The listing builds one solid part. Answer for the finished solid, in the listing's coordinates (mm). Round coordinates to 2 decimals unless told otherwise and drop trailing zeros. Order: outer loops, then holes, each group sorted by start corner. A loop starts at its lowest first (then second) coordinate and runs counter-clockwise, first axis right, second up. Notation, with made-up numbers: (13, 11) -> (36, 11) arc R8 ccw to (36, 17) -> close; hole circle Ø1 at (71.5, -1.75). An arc over 180 degrees is marked (long way). Return JSON: item names as keys, results as strings. Group by question number.
(1) Consider line 1 (X direction, y = 31.5, z = -1); line 2 (Y direction, x = 0.5, z = -31); line 3 (Y direction, x = 16.5, z = -3). Determine where each line is inside the solid, lowest interval first. Write a range as [from, to].
(2) The part is cut by section A-A (x = -11). Determine the outline of the cut face in (y, z), plus the area to 3 significant figures.
(3) The part is cut by section B-B (y = 24). Determine the outline of the cut face in (x, z), plus the area to 3 significant figures.
(4) The part is cut by section C-C (z = 33.5). Determine the outline of the cut face in (x, y).
(5) The part is cut by section D-D (y = -13.5). Determine the outline of the cut face in (x, z), plus the area to 3 significant figures.
(6) Each of these flat-tipped pins is pushed along its axis until it touches: pin 1 (24 mm diameter, centred on x = 1.5, z = 1.5, fed in from +Y); pin 2 (4 mm diameter, centred on x = -15.5, y = -4, fed in from -Z); pin 3 (1.5 mm diameter, centred on y = 39.5, z = 76, fed in from +X). Where does it stop, or does it pass through?
Autodesk Inventor part; units mm, degrees
ref_plane "Plano de trabalho1" through (0, 31, -25) normal (0, 0, 1) x (1, 0, 0)
ref_plane "YZ Plane" through (0, 0, 0) normal (1, 0, 0) x (0, 1, 0)
ref_plane "XZ Plane" through (0, 0, 0) normal (0, 1, 0) x (-1, 0, 0)
sketch "Esboço1" plane through (0, 0, 0) normal (0, 1, 0) x (-1, 0, 0)
  circle A0 centre (0, 0) radius 15
  dimension "d0" = 30
extrude "Extrusão1" add sketch "Esboço1" along normal blind 30
sketch "Esboço2" plane through (0, 30, 0) normal (0, 1, 0) x (1, 0, 0)
  circle A0 centre (0, 0) radius 2
  dimension "d3" = 4
extrude "Extrusão2" add sketch "Esboço2" along normal blind 1
sketch "Esboço3" plane through (0, 31, 0) normal (0, 1, 0) x (1, 0, 0)
  circle A0 centre (0, 0) radius 25
  dimension "d6" = 50
extrude "Extrusão3" add sketch "Esboço3" along normal blind 10
ref_plane "Plano de trabalho1" through (0, 31, -25) normal (0, 0, 1) x (1, 0, 0)
sketch "Esboço4" plane through (0, 31, -25) normal (0, 0, 1) x (1, 0, 0)
  line L0 (2, 0) -> (-2, 0)
  line L1 (0, 0) -> (0, 10)
  line L2 (25, 10) -> (-25, 10)
  circle A0 centre (0, 5) radius 2.5
  point P0 (0, -31)
  dimension "d9" = 5
extrude "Extrusão4" add sketch "Esboço4" along normal blind 80 and the other way blind 70
sketch "Esboço5" plane through (0, 0, 0) normal (1, 0, 0) x (0, 1, 0)
  line L0 (33.5, -95) -> (38.5, -95)
  line L1 (36, -95) -> (36, -105)
  line L2 (36, -95) -> (46, -95) construction
  line L3 (36, -105) -> (33.5, -95)
  line L4 (36, -95) -> (33.5, -95)
  point P0 (0, 0)
  dimension "d14" = 10
  dimension "d15" = 90
revolve "Revolução1" add sketch "Esboço5" angle 360 about axis through (0, 36, -95) along (0, 0, -1)
sketch "Esboço6" plane through (0, 0, 0) normal (1, 0, 0) x (0, 1, 0)
  line L0 (38.5, 55) -> (33.5, 55)
  line L1 (33.5, 25) -> (33.5, 55)
  line L2 (38.5, 25) -> (38.5, 55)
  line L3 (33.5, 55) -> (38.5, 55)
  line L4 (6, 113) -> (6, 101.4068)
  line L5 (6.7336, 98.7996) -> (33.5, 55)
  line L6 (8, 115) -> (84, 115)
  line L7 (86, 113) -> (86, 99.2532)
  line L8 (84.312, 95.5075) -> (38.5, 55)
  arc A0 (84.312, 95.5075) -> (86, 99.2532) centre (81, 99.2532) ccw
  arc A1 (6, 101.4068) -> (6.7336, 98.7996) centre (11, 101.4068) ccw
  arc A2 (8, 115) -> (6, 113) centre (8, 113) ccw
  arc A3 (86, 113) -> (84, 115) centre (84, 113) ccw
  point P0 (0, 0)
  point P1 (6, 115)
  point P2 (86, 115)
  point P3 (86, 97)
  dimension "d27" = 80
  dimension "d28" = 18
  dimension "d29" = 5
  dimension "d30" = 2
extrude "Extrusão5" add sketch "Esboço6" along normal mid plane 1.4
chamfer "Chanfro1" distance 1 angle 45 2 edges at (2, 34.5, 55) (-2.5, 36, 55)
sketch "Esboço7" plane through (0, 0, 0) normal (0, -1, 0) x (1, 0, 0)
  circle A0 centre (0, 0) radius 15
extrude "Extrusão6" add sketch "Esboço7" along normal blind 10
sketch "Esboço8" plane through (0, -10, 0) normal (0, -1, 0) x (1, 0, 0)
  circle A0 centre (0, 0) radius 1.5
  dimension "d39" = 3
extrude "Extrusão7" add sketch "Esboço8" along normal blind 25
thread "Rosca1"
properties part number "wind_vane"
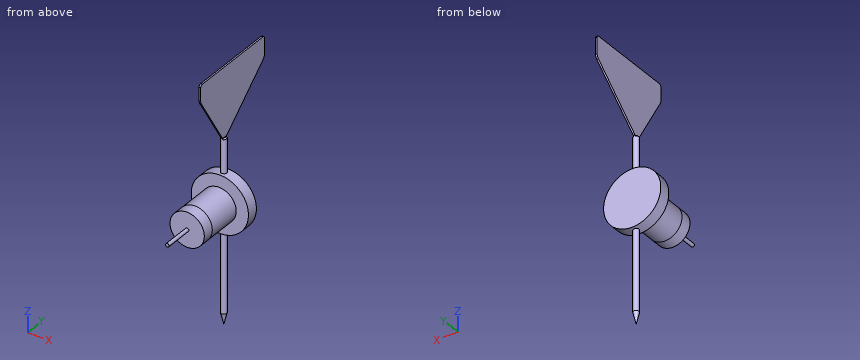
Answer below:
{
 "1": {"line 1": "x = [-24.98, 24.98]", "line 2": "y = [33.55, 38.45]", "line 3": "y = [31, 41]"},
 "2": {"outline": "(-10, -10.2) -> (30, -10.2) -> (30, 10.2) -> (-10, 10.2) -> close; (31, -22.45) -> (41, -22.45) -> (41, 22.45) -> (31, 22.45) -> close", "area": "1,260 mm²"},
 "3": {"outline": "circle Ø30 at (0, 0); (-0.7, 70.55) -> (0.7, 70.55) -> (0.7, 115) -> (-0.7, 115) -> close", "area": "769 mm²"},
 "4": {"outline": "circle Ø5 at (0, 36)"},
 "5": {"outline": "circle Ø3 at (0, 0)", "area": "7.07 mm²"},
 "6": {"pin 1": "stops at y = 41", "pin 2": "stops at z = -6.54", "pin 3": "stops at x = 0.7"}
}
